The listing builds one solid part. Answer for the finished solid, in the listing's coordinates (mm). A direction names the side the tool comes from. Give positions to 0.01 mm unless a question says otherwise; leave off trailing zeros. Loops run counter-clockwise (first coordinate to the right, second up) from the corner with the lowest first, then second, coordinate; pieces in that order, holes last. Notation, with made-up numbers: (53.5, 30.25) - (74.5, 30.25) arc R11 cw to (74.5, 40.25) - close; hole circle Ø11 at (74, 48.5). An arc over 180 degrees is marked (long way). One line per item, written item: value. Start each with the question number.
from build123d import *

# Parameters (mm, degrees)
SKETCH1_R         = 30
WHEEL_BLANK_DEPTH = 1.5
T_SLOT_DEPTH      = 2.5
CIRPATTERN1_COUNT = 12
SKETCH3_R         = 4
CENTER_HOLE_DEPTH = 6


with BuildPart() as part:
    # Sketch1 → Wheel Blank (new body)
    with BuildSketch(Plane(origin=(0, 0, 0), x_dir=(1, 0, 0), z_dir=(0, 1, 0))):
        Circle(SKETCH1_R)
    extrude(amount=WHEEL_BLANK_DEPTH)

    # Sketch2 → T-Slot (cut, through all)
    with BuildSketch(Plane(origin=(0, 0, 0), x_dir=(1, 0, 0), z_dir=(0, 1, 0))):
        with BuildLine():
            Line((-1.046984901, 29.981724811), (-0.994635656, 28.48263857))
            ThreePointArc((-0.994635656, 28.48263857), (-2.360033914, 28.402116821), (-3.719996478, 28.256178549))
            ThreePointArc((-3.719996478, 28.256178549), (-4.580915147, 27.134207496), (-3.458944094, 26.273288826))
            ThreePointArc((-3.458944094, 26.273288826), (0, 26.5), (3.458944094, 26.273288826))
            ThreePointArc((3.458944094, 26.273288826), (4.580915147, 27.134207496), (3.719996478, 28.256178549))
            ThreePointArc((3.719996478, 28.256178549), (2.360033914, 28.402116821), (0.994635656, 28.48263857))
            Line((0.994635656, 28.48263857), (1.046984901, 29.981724811))
            ThreePointArc((1.046984901, 29.981724811), (0, 30), (-1.046984901, 29.981724811))
        make_face()
    t_slot = extrude(amount=T_SLOT_DEPTH, mode=Mode.SUBTRACT)

    # CirPattern1: T-Slot ×12 about axis
    cirpattern1_axis = Axis((0, 0, 0), (0, 1, 0))
    for i in range(1, CIRPATTERN1_COUNT):
        add(t_slot.rotate(cirpattern1_axis, i * 360 / CIRPATTERN1_COUNT), mode=Mode.SUBTRACT)

    # Sketch3 → Center Hole (cut)
    with BuildSketch(Plane(origin=(0, 0, 0), x_dir=(1, 0, 0), z_dir=(0, 1, 0))):
        Circle(SKETCH3_R)
    extrude(amount=CENTER_HOLE_DEPTH, mode=Mode.SUBTRACT)


solid = part.part
1. A cutting plane is placed at C-C (z = 7.5). Determine the outline of the cut face in (x, y), plus the area to 3 significant figures.
2. A cutting plane is placed at D-D (x = 19). Determine the outline of the cut face in (y, z).
3. A flat-ended cylindrical pin translates along its axis: pin 1 (5 mm diameter, centred on x = 0, z = 0, fed in from -Y). Find the tip coordinate at first contact, or state that the pin passes through.
4. A cutting plane is placed at A-A (x = 0). Determine the outline of the cut face in (y, z).
5. For faces 1 (the cylindrical face through (-29.002, 0.74, 7.672)), 2 (the cylindrical face through (-22.974, 0.74, -13.208)), determine the directions among +Z, -Z, +X, -X, +Y, -Y from which every point of the face is accessible in a straight line to the end or side of a thin tool.
6. Find the intervals of material crossed by L1, parallel to Z at x = 0, y = 0.4; L2, parallel to Z at x = 23, y = 0.1; L3, parallel to Z at x = -3, y = 1.2, in increasing order. Write a range as [from, to].
7. A cutting plane is placed at B-B (z = 0). Determine the outline of the cut face in (x, y).
8. Determine the mould class of faces 3 (the flat face through (0, 1.5, 6)), 4 (the cylindrical face through (7.86, 0.74, -28.95)), 5 (the cylindrical face through (-17.52, 0.74, 21.19)), 6 (the cylindrical face through (-16.261, 0.74, 23.406)) for opening direction Z: released by +Z, released by -Z, zero draft, split by the parting line, or undercut.
Results below:
1. outline: (-29.05, 0) - (29.05, 0) - (29.05, 1.5) - (-29.05, 1.5) - close
1. area: 87.1 mm^2
2. outline: (0, -23.22) - (1.5, -23.22) - (1.5, 23.22) - (0, 23.22) - close
3. pin 1: passes through
4. outline: (0, -26.5) - (1.5, -26.5) - (1.5, -4) - (0, -4) - close; (0, 4) - (1.5, 4) - (1.5, 26.5) - (0, 26.5) - close
5. face 1: +Z, -X, +Y, -Y
5. face 2: +Y, -Y
6. L1: z = [-26.5, -4], [4, 26.5]
6. L2: z = [-19.26, -16.83], [-13.16, 13.16], [16.83, 19.26]
6. L3: z = [-29.85, -28.34], [-26.33, -2.65], [2.65, 26.33], [28.34, 29.85]
7. outline: (-26.5, 0) - (-4, 0) - (-4, 1.5) - (-26.5, 1.5) - close; (4, 0) - (26.5, 0) - (26.5, 1.5) - (4, 1.5) - close
8. face 3: zero draft
8. face 4: released by -Z
8. face 5: undercut
8. face 6: undercut
